Autodesk Inventor part; units mm, degrees
ref_plane "YZ Plane" through (0, 0, 0) normal (1, 0, 0) x (0, 1, 0)
ref_plane "XZ Plane" through (0, 0, 0) normal (0, 1, 0) x (-1, 0, 0)
ref_plane "XY Plane" through (0, 0, 0) normal (0, 0, 1) x (1, 0, 0)
sketch "Sketch1" plane through (0, 0, 0) normal (0, 0, 1) x (1, 0, 0)
  line L0 (0, 0) -> (-17, 0)
  line L1 (-17, 0) -> (-17, -10)
  line L2 (-17, -10) -> (0, -10)
  line L3 (0, -10) -> (0, 0)
  line L4 (-17, 0) -> (-14, 0)
  line L5 (-14, 0) -> (-14, 6)
  line L6 (-14, 6) -> (-17, 6)
  line L7 (-17, 6) -> (-17, 0)
  line L8 (-14, 4) -> (-15, 4)
  line L9 (-15, 4) -> (-15, 2)
  line L10 (-15, 2) -> (-14, 2)
  line L11 (-14, 2) -> (-14, 4)
  line L12 (0, 0) -> (-3, 0)
  line L13 (-3, 0) -> (-3, 6)
  line L14 (-3, 6) -> (0, 6)
  line L15 (0, 6) -> (0, 0)
  line L16 (-3, 4) -> (-2, 4)
  line L17 (-2, 4) -> (-2, 2)
  line L18 (-2, 2) -> (-3, 2)
  line L19 (-3, 2) -> (-3, 4)
  dimension "d1" = 10
  dimension "d10" = 13
  dimension "d11" = 2
  dimension "d12" = 2
  dimension "d13" = 2
  dimension "d14" = 2
  dimension "d15" = 2
  dimension "d16" = 1
  dimension "d17" = 1
extrude "Extrusion1" add sketch "Sketch1" along normal blind 15 contours L3 L2 L1 L0 | L0 L13 L18 L17 L16 L14 L15 | L0 L7 L6 L5 L8 L9 L10
sketch "Sketch2" plane through (0, 0, 15) normal (0, 0, 1) x (1, 0, 0)
  circle A0 centre (-8.5, -5) radius 1.25
  line L0 (0, 0) -> (-14, 0)
  point P0 (-17, 0)
  point P1 (-8.5, 0)
  dimension "d4" = 5
  dimension "d5" = 2.5
sketch "Sketch4" plane through (0, 0, 0) normal (0, 0, -1) x (-1, 0, 0)
  line L0 (0, -10) -> (0, 6)
  line L1 (17, 6) -> (17, -10)
  line L2 (0, -10) -> (17, -10)
  line L3 (17, -10) -> (17, 6)
  line L4 (17, 6) -> (0, 6)
  line L5 (0, 6) -> (0, -10)
  point P0 (0, 0)
  point P1 (0, 6)
extrude "Extrusion3" add sketch "Sketch4" along normal blind 2
extrude "Extrusion4" cut sketch "Sketch2" against normal through all
equation "\"d15\" = d11"
equation "\"d16\" = d17"
properties part number "usb port mount"
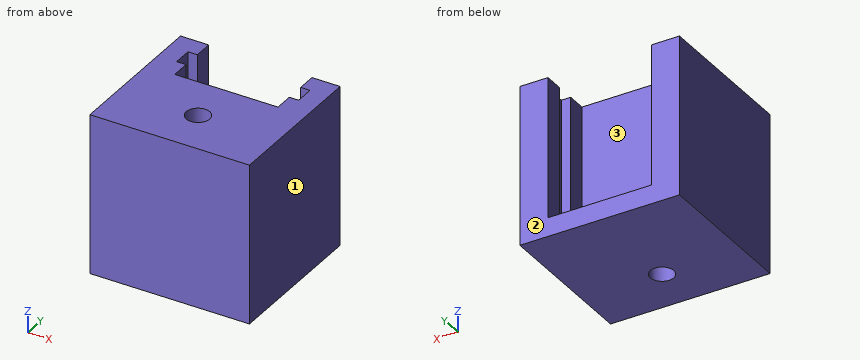
Verification items for the finished model (mm, model axes). Face numbers are marked on the shaded views. Coordinates: 2 decimals unless noted, no trailing zeros. Order: outer loops, then holes, each group sorted by start corner. A loop starts at its lowest first (then second) coordinate and runs counter-clockwise, first axis right, second up. Notation, with made-up numbers: (89, -23.5) -> (130, -23.5) arc R24 cw to (130, -7.5) -> close; hole circle Ø2 at (83, -35). An arc over 180 degrees is marked (long way). Put each result on its own line as item: value. Start each with the question number.
1) Cross-section at A-A (x = -8.5). Enter the section's corners in (y, z), plus the area to 4 significant figures.
2) Material ranges on L1, parallel to X at y = 3.25, z = 11; L2, parallel to Y at x = -8.5, z = 6.25; L3, parallel to Z at x = -6.25, y = 1.75, recorded low to high.
3) Cross-section at D-D (y = 1.25). Enter the section's corners in (x, z).
4) Go/stop test with flat-tipped pins: pin 1 (6.5 mm diameter, centred on x = -9, y = 3.5, fed in from +Z); pin 2 (1 mm diameter, centred on x = -12.5, z = 2.5, fed in from +Y). Record where each tip stops, or that it passes through.
5) Cross-section at B-B (z = 9.5). Enter the section's corners in (x, y).
6) Release check for a two-part mould opening along X. For the marked faces 1, 2 and 3 record: pulls with the +X half, pulls with the -X half, needs draft (parallel to the pull), parting line crosses it, or undercut.
7) Cross-section at C-C (y = -4.5). Enter the section's corners in (x, z), plus the area to 3 significant figures.
Geometry check:
1. outline: (-10, -2) -> (-6.25, -2) -> (-6.25, 15) -> (-10, 15) -> close; (-3.75, -2) -> (6, -2) -> (6, 0) -> (0, 0) -> (0, 15) -> (-3.75, 15) -> close
1. area: 139.5 mm^2
2. L1: x = -17 to -15, -2 to 0
2. L2: y = -10 to -6.25, -3.75 to 0
2. L3: z = -2 to 0
3. outline: (-17, -2) -> (0, -2) -> (0, 15) -> (-3, 15) -> (-3, 0) -> (-14, 0) -> (-14, 15) -> (-17, 15) -> close
4. pin 1: stops at z = 0
4. pin 2: stops at y = 0
5. outline: (-17, -10) -> (0, -10) -> (0, 6) -> (-3, 6) -> (-3, 4) -> (-2, 4) -> (-2, 2) -> (-3, 2) -> (-3, 0) -> (-14, 0) -> (-14, 2) -> (-15, 2) -> (-15, 4) -> (-14, 4) -> (-14, 6) -> (-17, 6) -> close; hole circle Ø2.5 at (-8.5, -5)
6. face 1: pulls with the +X half
6. face 2: needs draft
6. face 3: undercut
7. outline: (-17, -2) -> (-9.65, -2) -> (-9.65, 15) -> (-17, 15) -> close; (-7.35, -2) -> (0, -2) -> (0, 15) -> (-7.35, 15) -> close
7. area: 250 mm^2
